from build123d import *

# Parameters (mm, degrees)
F0_R     = 101.6
F1_DEPTH = 25.4
F2_T     = -2.54


# Not quite as in the source:
# - a fillet or chamfer that OpenCascade refuses, or shapes differently, is made with other operations: its cross-section is extruded or revolved along the edge and cut away or added


with BuildPart() as f1:
    # F0 (on Front) → F1 (new body)
    with BuildSketch(Plane.XZ):
        Circle(F0_R)
    extrude(amount=F1_DEPTH)

    # F2
    f2_openings = [f1.faces().sort_by_distance(p)[0] for p in [
        (0, 0, 0),
    ]]
    offset(amount=F2_T, openings=f2_openings)

    # F3: fillet of radius 5.08 on 2 edges, made by hand

    # F3_s1 → F3_t2 (revolve, cut)
    with BuildSketch(Plane.XY):
        with BuildLine():
            ThreePointArc((101.6, -20.32), (100.1121024484, -23.9121024484), (96.52, -25.4))
            Line((96.52, -25.4), (101.6, -25.4))
            Line((101.6, -25.4), (101.6, -20.32))
        make_face()
    revolve(axis=Axis((0, -25.4, 0), (0, -1, 0)), mode=Mode.SUBTRACT)

    # F3_s3 → F3_t4 (revolve, cut)
    with BuildSketch(Plane.XY):
        with BuildLine():
            ThreePointArc((101.6, -4.3994090512), (100.9194090512, -1.8594090512), (99.06, 0))
            Line((99.06, 0), (101.6, 0))
            Line((101.6, 0), (101.6, -4.3994090512))
        make_face()
    revolve(axis=Axis((0, 0, 0), (0, -1, 0)), mode=Mode.SUBTRACT)


solid = f1.part
Build history of the part. All positions in model axes, mm. Round coordinates to 2 decimals unless told otherwise and drop trailing zeros. Loops run counter-clockwise (first coordinate to the right, second up) from the corner with the lowest first, then second, coordinate; pieces in that order, holes last. Notation, with made-up numbers: (19, -34.5) -> (52, -34.5) arc R12 cw to (52, -29.5) -> close; hole circle Ø11 at (2.5, 47). An arc over 180 degrees is marked (long way). Answer in a Markdown table with one row per item.
Item 1: Saw through at A-A (x = 0). Write the cut outline in (y, z).
Answers below:
| item | result |
|---|---|
| outline | (-25.4, -96.52) arc R5.08 ccw to (-20.32, -101.6) -> (-4.4, -101.6) arc R5.08 ccw to (0, -99.06) -> (-22.86, -99.06) -> (-22.86, 99.06) -> (0, 99.06) arc R5.08 ccw to (-4.4, 101.6) -> (-20.32, 101.6) arc R5.08 ccw to (-25.4, 96.52) -> close |
Item 2: Saw through at B-B (y = -10.75). Write the cut outline in (x, z), and give its area (3 significant figures).
Answers below:
| item | result |
|---|---|
| outline | circle Ø203.2 at (0, 0); hole circle Ø198.12 at (0, 0) |
| area | 1,600 mm² |
Item 3: Saw through at C-C (z = 0). Write the cut outline in (x, y).
Answers below:
| item | result |
|---|---|
| outline | (-101.6, -20.32) arc R5.08 ccw to (-96.52, -25.4) -> (96.52, -25.4) arc R5.08 ccw to (101.6, -20.32) -> (101.6, -4.4) arc R5.08 ccw to (99.06, 0) -> (99.06, -22.86) -> (-99.06, -22.86) -> (-99.06, 0) arc R5.08 ccw to (-101.6, -4.4) -> close |
Item 4: Mould opens along X. For faces 1 (the cylindrical face through (-22.025, -12.248, -99.184)), 2 (the flat face through (-1, -25.4, 1)), 3 (the flat face through (-1, -22.86, 1)) say: +X half, -X half, draft (parallel to the pull), parting line (faces both ways), or undercut.
Answers below:
| item | result |
|---|---|
| face 1 | parting line |
| face 2 | draft |
| face 3 | undercut |
Item 5: Drill centre lines: L1, parallel to Z at x = -3, y = -14; L2, parallel to Z at x = 0, y = -6.75; L3, parallel to Y at x = -44.5, z = -73. Where is each one in solid material? Low to high. Write a range as [from, to].
Answers below:
| item | result |
|---|---|
| L1 | z = [-101.56, -99.01], [99.01, 101.56] |
| L2 | z = [-101.6, -99.06], [99.06, 101.6] |
| L3 | y = [-25.4, -22.86] |
Item 6: Pin check, flat tips, straight feed: pin 1 (1.5 mm diameter, centred on y = -4, z = -80, fed in from -X); pin 2 (8 mm diameter, centred on x = -43.5, y = -15, fed in from +Z); pin 3 (1 mm diameter, centred on y = -14, z = 5, fed in from -X). Stop position of each tip, or through.
Answers below:
| item | result |
|---|---|
| pin 1 | stops at x = -63.56 |
| pin 2 | stops at z = 93.61 |
| pin 3 | stops at x = -101.5 |
